Check sheet for the modelled part. Datum: model origin and axes. Units: mm. Face numbers are marked on the shaded views. A direction names the side the tool comes from. Round coordinates to 2 decimals unless told otherwise and drop trailing zeros. Write each loop counter-clockwise with the first axis right and the second up, starting at its lowest first coordinate (ties: lowest second). Pieces come first, ordered by that corner, then holes.
Item 1: Material ranges on line 1 (Y direction, x = 4, z = 17.25); line 2 (X direction, y = -0.75, z = 10), recorded low to high.
Item 2: Release check for a two-part mould opening along Z. For the marked faces 1, 2, 3 and 4 record: +Z half, -Z half, draft (parallel to the pull), parting line (faces both ways), or undercut.
Item 3: Cross-section at B-B on x = 10. Enter the section's corners in (y, z).
Item 4: Cross-section at A-A on y = 25. Enter the section's corners in (x, z).
Item 5: Cross-section at C-C on z = 10. Enter the section's corners in (x, y).
Item 6: Cross-section at D-D on z = 13.25. Enter the section's corners in (x, y), plus the area to 3 significant figures.
Item 7: Go/stop test with flat-tipped pins: pin 1 Ø1 at (x, z) = (1.5, 2) entering from +Y; pin 2 Ø1.5 at (y, z) = (42, 14.5) entering from +X; pin 3 Ø7.5 at (x, z) = (10, 10) entering from +Y. Record where each tip stops, or that it passes through.
Item 8: Tool access check on the marked faces 5, 6 and 7. Record the directions out of +Z, -Z, +X, -X, +Y, -Y that give a thin tool (end or side, any length) a straight path to the whole face; none if there is none.
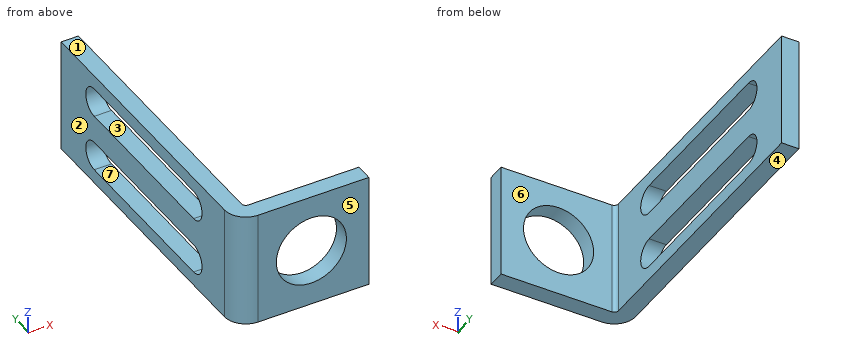
from build123d import *

# Parameters (mm, degrees)
BASE_FLANGE1_DEPTH = 20
CUT_EXTRUDE1_REACH = 59.446
SKETCH6_R          = 6.1
CUT_EXTRUDE2_REACH = 59.446


# Sheet-metal steps are written as plain solids
with BuildPart() as part:
    # Sketch1 → Base-Flange1 (new body)
    with BuildSketch(Plane.XY):
        with BuildLine():
            Line((0, 50), (0, 0.7366))
            ThreePointArc((0, 0.7366), (0.215745145, 0.215745145), (0.7366, 0))
            Line((0.7366, 0), (20, 0))
            Line((20, 0), (20, -3))
            Line((20, -3), (0.7366, -3))
            ThreePointArc((0.7366, -3), (-1.905575199, -1.905575199), (-3, 0.7366))
            Line((-3, 0.7366), (-3, 50))
            Line((-3, 50), (0, 50))
        make_face()
    extrude(amount=BASE_FLANGE1_DEPTH)

    # Sketch6 → Cut-Extrude1 (cut, up to next)
    with BuildSketch(Plane(origin=(0, 0, 0), x_dir=(1, 0, 0), z_dir=(0, 1, 0)), mode=Mode.PRIVATE) as cut_extrude1_sk1:
        with Locations(Location((10, -10, 0), (0, 0, 270))):
            Circle(SKETCH6_R)
    cut_extrude1_tool1 = extrude(cut_extrude1_sk1.sketch, amount=-CUT_EXTRUDE1_REACH, mode=Mode.PRIVATE) & part.part
    add(cut_extrude1_tool1.solids().sort_by_distance((10, 0, 10))[0], mode=Mode.SUBTRACT)

    # Sketch7 → Cut-Extrude2 (cut, up to next)
    with BuildSketch(Plane(origin=(0, 0, 0), x_dir=(0, 0, -1), z_dir=(1, 0, 0)), mode=Mode.PRIVATE) as cut_extrude2_sk1:
        with BuildLine():
            Line((-12.45, 40), (-12.45, 10))
            ThreePointArc((-12.45, 10), (-15, 7.45), (-17.55, 10))
            Line((-17.55, 10), (-17.55, 40))
            ThreePointArc((-17.55, 40), (-15, 42.55), (-12.45, 40))
        make_face()
    cut_extrude2_tool1 = extrude(cut_extrude2_sk1.sketch, amount=-CUT_EXTRUDE2_REACH, mode=Mode.PRIVATE) & part.part
    # Sketch7 → Cut-Extrude2 (cut, up to next)
    with BuildSketch(Plane(origin=(0, 0, 0), x_dir=(0, 0, -1), z_dir=(1, 0, 0)), mode=Mode.PRIVATE) as cut_extrude2_sk2:
        with BuildLine():
            Line((-2.45, 40), (-2.45, 10))
            ThreePointArc((-2.45, 10), (-5, 7.45), (-7.55, 10))
            Line((-7.55, 10), (-7.55, 40))
            ThreePointArc((-7.55, 40), (-5, 42.55), (-2.45, 40))
        make_face()
    cut_extrude2_tool2 = extrude(cut_extrude2_sk2.sketch, amount=-CUT_EXTRUDE2_REACH, mode=Mode.PRIVATE) & part.part
    add(cut_extrude2_tool1.solids().sort_by_distance((0, 25, 15))[0], mode=Mode.SUBTRACT)
    add(cut_extrude2_tool2.solids().sort_by_distance((0, 25, 5))[0], mode=Mode.SUBTRACT)


solid = part.part
Response values:
1. line 1: y = -3 to 0
1. line 2: x = -2.69 to 3.9, 16.1 to 20
2. face 1: +Z half
2. face 2: draft
2. face 3: undercut
2. face 4: -Z half
3. outline: (-3, 0) - (0, 0) - (0, 3.9) - (-3, 3.9) - close; (-3, 16.1) - (0, 16.1) - (0, 20) - (-3, 20) - close
4. outline: (-3, 0) - (0, 0) - (0, 2.45) - (-3, 2.45) - close; (-3, 7.55) - (0, 7.55) - (0, 12.45) - (-3, 12.45) - close; (-3, 17.55) - (0, 17.55) - (0, 20) - (-3, 20) - close
5. outline: (-3, 0.74) arc R3.74 ccw to (0.74, -3) - (3.9, -3) - (3.9, 0) - (0.74, 0) arc R0.74 cw to (0, 0.74) - (0, 50) - (-3, 50) - close; (16.1, -3) - (20, -3) - (20, 0) - (16.1, 0) - close
6. outline: (-3, 0.74) arc R3.74 ccw to (0.74, -3) - (4.84, -3) - (4.84, 0) - (0.74, 0) arc R0.74 cw to (0, 0.74) - (0, 8.15) - (-3, 8.15) - close; (-3, 41.85) - (0, 41.85) - (0, 50) - (-3, 50) - close; (15.16, -3) - (20, -3) - (20, 0) - (15.16, 0) - close
6. area: 84.0 mm2
7. pin 1: stops at y = 0
7. pin 2: stops at x = 0
7. pin 3: passes through
8. face 5: +Z, -Z, +X, -X, -Y
8. face 6: +Z, -Z, +X, +Y
8. face 7: +X, -X
